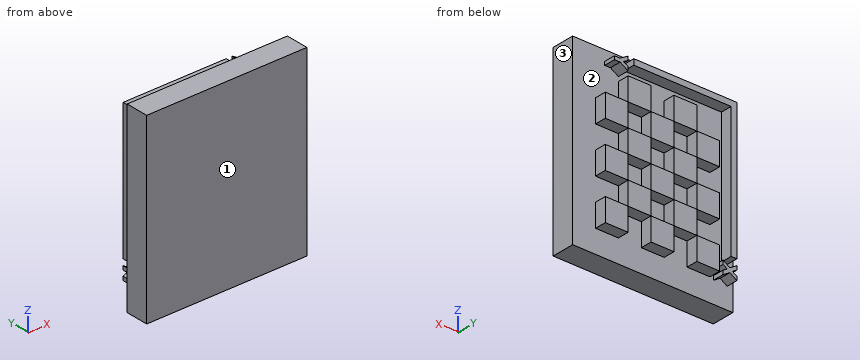
Autodesk Inventor part; units mm, degrees
ref_plane "YZ Plane" through (0, 0, 0) normal (1, 0, 0) x (0, 1, 0)
ref_plane "XZ Plane" through (0, 0, 0) normal (0, 1, 0) x (-1, 0, 0)
ref_plane "XY Plane" through (0, 0, 0) normal (0, 0, 1) x (1, 0, 0)
sketch "Sketch1" plane through (0, 0, 0) normal (0, 1, 0) x (-1, 0, 0)
  line L0 (70, 80) -> (-70, 80)
  line L1 (-70, 80) -> (-70, -80)
  line L2 (-70, -80) -> (70, -80)
  line L3 (70, -80) -> (70, 80)
  point P0 (0, 0)
  dimension "d0" = 140
  dimension "d1" = 160
  dimension "d4" = 70
  dimension "d5" = 80
extrude "Extrusion1" add sketch "Sketch1" along normal blind 20
sketch "Sketch2" plane through (0, 20, 0) normal (0, 1, 0) x (1, 0, 0)
  line L0 (50, 60) -> (-50, 60)
  line L1 (-50, 60) -> (-50, -60)
  line L2 (-50, -60) -> (50, -60)
  line L3 (50, -60) -> (50, 60)
  line L4 (50, 60) -> (-50, -60) construction
  line L5 (-50, 60) -> (50, -60) construction
  point P0 (0, 0)
  dimension "d8" = 100
  dimension "d9" = 120
extrude "Extrusion2" add sketch "Sketch2" along normal blind 10
sketch "Sketch3" plane through (0, 30, 0) normal (0, 1, 0) x (1, 0, 0)
  line L0 (-50, 60) -> (-50, -60)
  line L1 (-50, -60) -> (-30, -60)
  line L2 (-30, -60) -> (-30, -40)
  line L3 (-30, -40) -> (-50, -40)
  line L4 (-50, -40) -> (-50, -60)
  line L5 (-10, -60) -> (10, -60)
  line L6 (10, -60) -> (10, -40)
  line L7 (10, -40) -> (-10, -40)
  line L8 (-10, -40) -> (-10, -60)
  line L9 (10, -40) -> (30, -40)
  line L10 (30, -40) -> (30, -20)
  line L11 (30, -20) -> (10, -20)
  line L12 (10, -20) -> (10, -40)
  line L13 (-30, -40) -> (-10, -40)
  line L14 (-10, -40) -> (-10, -20)
  line L15 (-10, -20) -> (-30, -20)
  line L16 (-30, -20) -> (-30, -40)
  line L17 (-50, -60) -> (50, -60)
  line L18 (-53.5785, -189.3047) -> (-33.5785, -189.3047)
  line L19 (-33.5785, -189.3047) -> (-33.5785, -169.3047)
  line L20 (-33.5785, -169.3047) -> (-53.5785, -169.3047)
  line L21 (-53.5785, -169.3047) -> (-53.5785, -189.3047)
  line L22 (-50, -20) -> (-30, -20)
  line L23 (-30, -20) -> (-30, 0)
  line L24 (-30, 0) -> (-50, 0)
  line L25 (-50, 0) -> (-50, -20)
  line L26 (-10, -20) -> (10, -20)
  line L27 (10, -20) -> (10, 0)
  line L28 (10, 0) -> (-10, 0)
  line L29 (-10, 0) -> (-10, -20)
  line L30 (10, 40) -> (30, 40)
  line L31 (30, 40) -> (30, 60)
  line L32 (30, 60) -> (10, 60)
  line L33 (10, 60) -> (10, 40)
  line L34 (-10, 20) -> (-30, 20)
  line L35 (-30, 0) -> (-10, 0)
  line L36 (-30, 20) -> (-30, 0)
  line L37 (-10, 0) -> (-10, 20)
  line L38 (10, 40) -> (-10, 40)
  line L39 (-10, 20) -> (10, 20)
  line L40 (-10, 40) -> (-10, 20)
  line L41 (10, 20) -> (10, 40)
  line L42 (30, 20) -> (10, 20)
  line L43 (10, 0) -> (30, 0)
  line L44 (10, 20) -> (10, 0)
  line L45 (30, 0) -> (30, 20)
  line L46 (-10, 60) -> (-30, 60)
  line L47 (-30, 40) -> (-10, 40)
  line L48 (-30, 60) -> (-30, 40)
  line L49 (-10, 40) -> (-10, 60)
  line L50 (-30, 40) -> (-50, 40)
  line L51 (-50, 20) -> (-30, 20)
  line L52 (-50, 40) -> (-50, 20)
  line L53 (-30, 20) -> (-30, 40)
  line L54 (30, 20) -> (50, 20)
  line L55 (50, 20) -> (50, 40)
  line L56 (50, 40) -> (30, 40)
  line L57 (30, 40) -> (30, 20)
  line L58 (30, -20) -> (50, -20)
  line L59 (50, -20) -> (50, 0)
  line L60 (50, 0) -> (30, 0)
  line L61 (30, 0) -> (30, -20)
  line L62 (30, -60) -> (50, -60)
  line L63 (50, -60) -> (50, -40)
  line L64 (50, -40) -> (30, -40)
  line L65 (30, -40) -> (30, -60)
  dimension "d12" = 20
  dimension "d13" = 20
  dimension "d14" = 20
  dimension "d15" = 20
  dimension "d17" = 20
  dimension "d18" = 20
  dimension "d19" = 20
  dimension "d21" = 20
  dimension "d22" = 20
  dimension "d25" = 20
  dimension "d26" = 20
  dimension "d27" = 20
  dimension "d28" = 20
  dimension "d30" = 20
  dimension "d31" = 20
  dimension "d33" = 20
  dimension "d34" = 20
  dimension "d36" = 20
  dimension "d37" = 20
  dimension "d39" = 20
  dimension "d40" = 20
  dimension "d42" = 20
  dimension "d43" = 20
  dimension "d45" = 20
  dimension "d46" = 20
  dimension "d48" = 20
  dimension "d49" = 20
  dimension "d77" = 20
  dimension "d78" = 20
  dimension "d80" = 20
  dimension "d81" = 20
  dimension "d83" = 20
  dimension "d84" = 20
extrude "Extrusion5" cut sketch "Sketch3" against normal blind 10 contours L50 L53 L51 L0 | L48 L46 L49 L47 | L24 L23 L22 L0 | L34 L37 L35 L36 | L38 L41 L39 L40 | L33 L32 L31 L30 | L3 L2 L1 L0 | L15 L14 L13 L16 | L28 L27 L26 L29 | L42 L45 L43 L44 | L56 L55 L54 L57 | L7 L6 L5 L8 | L11 L10 L9 L12 | L60 L59 L58 L61 | L64 L63 L17 L65
sketch "Sketch4" plane through (0, 20, 0) normal (0, 1, 0) x (1, 0, 0)
  line L0 (-65, -75) -> (-65, 45)
  line L1 (-65, 45) -> (-60, 45)
  line L2 (-60, 45) -> (-60, -70)
  line L3 (-60, -70) -> (25, -70)
  line L4 (25, -70) -> (25, -75)
  line L5 (25, -75) -> (-65, -75)
  line L6 (-70, -80) -> (70, -80)
  line L7 (-70, 80) -> (-70, -80)
  line L8 (-53.0136, 61.5997) -> (-53.0136, 50) construction
  line L9 (-53.0136, 50) -> (-65.2641, 50) construction
  line L10 (-65.2641, 50) -> (-65.2641, 61.5997) construction
  line L11 (-65.2641, 61.5997) -> (-53.0136, 61.5997) construction
  line L12 (30, -75) -> (30, -63.5159) construction
  line L13 (30, -63.5159) -> (34.1954, -63.5159) construction
  line L14 (34.1954, -63.5159) -> (34.1954, -75) construction
  line L15 (34.1954, -75) -> (30, -75) construction
  line L16 (-65.0136, 50.2026) -> (-65.0136, 53.684)
  line L17 (-65.0136, 53.684) -> (-61.1919, 55.9984)
  line L18 (-61.1919, 55.9984) -> (-65.0136, 58.3615)
  line L19 (-65.0136, 58.3615) -> (-65.0136, 61.697)
  line L20 (-65.0136, 61.697) -> (-58.9747, 57.7975)
  line L21 (-58.9747, 57.7975) -> (-53.0136, 61.5414)
  line L22 (-53.0136, 61.5414) -> (-53.0136, 58.06)
  line L23 (-53.0136, 58.06) -> (-56.6408, 55.8915)
  line L24 (-56.6408, 55.8915) -> (-53.0136, 53.6646)
  line L25 (-53.0136, 53.6646) -> (-53.0136, 50.3291)
  line L26 (-53.0136, 50.3291) -> (-58.8483, 54.0924)
  line L27 (-58.8483, 54.0924) -> (-65.0136, 50.2026)
  line L28 (30, -63.778) -> (36.9919, -67.9206)
  line L29 (36.9919, -67.9206) -> (42, -67.9206)
  line L30 (42, -67.9206) -> (42, -70.9352)
  line L31 (42, -70.9352) -> (37.1378, -70.9352)
  line L32 (37.1378, -70.9352) -> (30, -75.1459)
  line L33 (30, -75.1459) -> (30, -71.7131)
  line L34 (30, -71.7131) -> (34.2788, -69.3695)
  line L35 (34.2788, -69.3695) -> (30, -67.1037)
  line L36 (30, -67.1037) -> (30, -63.778)
  point P0 (0, 0)
  point P1 (-62.5, 45)
  point P2 (-58.8748, 54.3197)
  point P3 (25, -72.5)
  point P4 (28.8521, -69.3123)
  point P5 (28.8521, -69.3123)
  dimension "d53" = 5
  dimension "d54" = 5
  dimension "d55" = 5
  dimension "d56" = 5
  dimension "d57" = 120
  dimension "d58" = 90
  dimension "d63" = 12.2505
  dimension "d73" = 5
  dimension "d88" = 5
  dimension "d90" = 5
extrude "Extrusion4" add sketch "Sketch4" along normal blind 10
equation "\"d12\" = cell"
equation "\"d13\" = cell"
equation "\"d14\" = d16"
equation "\"d15\" = d16"
equation "\"d17\" = cell"
equation "\"d18\" = d20"
equation "\"d19\" = d20"
equation "\"d21\" = d23"
equation "\"d22\" = d23"
equation "\"d25\" = cell"
equation "\"d26\" = cell"
equation "\"d27\" = d29"
equation "\"d28\" = d29"
equation "\"d30\" = d32"
equation "\"d31\" = d32"
equation "\"d33\" = d35"
equation "\"d34\" = d35"
equation "\"d36\" = d38"
equation "\"d37\" = d38"
equation "\"d39\" = d41"
equation "\"d40\" = d41"
equation "\"d42\" = d44"
equation "\"d43\" = d44"
equation "\"d45\" = d47"
equation "\"d46\" = d47"
equation "\"d48\" = d50"
equation "\"d49\" = d50"
equation "\"cell\" = 20"
equation "\"d16\" = 20"
equation "\"d20\" = 20"
equation "\"d23\" = 20"
equation "\"d29\" = 20"
equation "\"d32\" = 20"
equation "\"d35\" = 20"
equation "\"d38\" = 20"
equation "\"d41\" = 20"
equation "\"d44\" = 20"
equation "\"d47\" = 20"
equation "\"d50\" = 20"
properties part number "3D_Grid"
For this review, take the finished solid that the model builds, in its own axes (mm). Face numbers are marked on the shaded views. Round coordinates to 2 decimals unless told otherwise and drop trailing zeros. Write each loop counter-clockwise with the first axis right and the second up, starting at its lowest first coordinate (ties: lowest second). Pieces come first, ordered by that corner, then holes. Notation, with made-up numbers: (28, 0.25) - (42, 0.25) arc R4 ccw to (42, 4.25) - close; hole circle Ø9 at (-13.5, -13.75). An arc over 180 degrees is marked (long way). Use a Markdown table: item, result.
Q1. We need section D-D (z = 8). Give the boundary of the cut face in (x, y), plus the area to 3 significant figures.
Derived:
| item | result |
|---|---|
| outline | (-70, 0) - (70, 0) - (70, 20) - (30, 20) - (30, 30) - (10, 30) - (10, 20) - (-10, 20) - (-10, 30) - (-30, 30) - (-30, 20) - (-60, 20) - (-60, 30) - (-65, 30) - (-65, 20) - (-70, 20) - close |
| area | 3,250 mm2 |
Q2. Clearance check with flat-ended pins moving along their axes: pin 1 (8 mm diameter, centred on x = -17, y = 23, fed in from +Z); pin 2 (2 mm diameter, centred on x = 4.5, z = -32.5, fed in from +Y); pin 3 (2.5 mm diameter, centred on y = 25.5, z = 65.5, fed in from -X); pin 4 (2.5 mm diameter, centred on y = 26.5, z = 71.5, fed in from +X). State where each tip first meets the part, or that it passes through.
Derived:
| item | result |
|---|---|
| pin 1 | stops at z = 80 |
| pin 2 | stops at y = 20 |
| pin 3 | stops at x = -65 |
| pin 4 | stops at x = 42 |
Q3. We need section A-A (z = 33.5). Give the boundary of the cut face in (x, y), plus the area to 3 significant figures.
Derived:
| item | result |
|---|---|
| outline | (-70, 0) - (70, 0) - (70, 20) - (50, 20) - (50, 30) - (30, 30) - (30, 20) - (10, 20) - (10, 30) - (-10, 30) - (-10, 20) - (-30, 20) - (-30, 30) - (-50, 30) - (-50, 20) - (-60, 20) - (-60, 30) - (-65, 30) - (-65, 20) - (-70, 20) - close |
| area | 3,450 mm2 |
Q4. Wall thickness on line 1 along Z through (x, y) = (-34.5, 25.5); line 2 along X through (y, z) = (25.5, 16.5); line 3 along Z through (x, y) = (48, 20.5): over which ranges is each line inside the solid? List them lowest first.
Derived:
| item | result |
|---|---|
| line 1 | z = -60 to -40, -20 to 0, 20 to 40, 70 to 75 |
| line 2 | x = -65 to -60, -30 to -10, 10 to 30 |
| line 3 | z = -60 to -40, -20 to 0, 20 to 40 |
Q5. We need section B-B (x = -38). Give the boundary of the cut face in (y, z).
Derived:
| item | result |
|---|---|
| outline | (0, -80) - (20, -80) - (20, -60) - (30, -60) - (30, -40) - (20, -40) - (20, -20) - (30, -20) - (30, 0) - (20, 0) - (20, 20) - (30, 20) - (30, 40) - (20, 40) - (20, 70) - (30, 70) - (30, 75) - (20, 75) - (20, 80) - (0, 80) - close |
Q6. The part is to be moulded in two halves that separate along X. For the marked faces 1, 2 and 3, say which applies: pulls with the +X half, pulls with the -X half, needs draft (parallel to the pull), parting line crosses it, or undercut.
Derived:
| item | result |
|---|---|
| face 1 | needs draft |
| face 2 | undercut |
| face 3 | pulls with the +X half |
